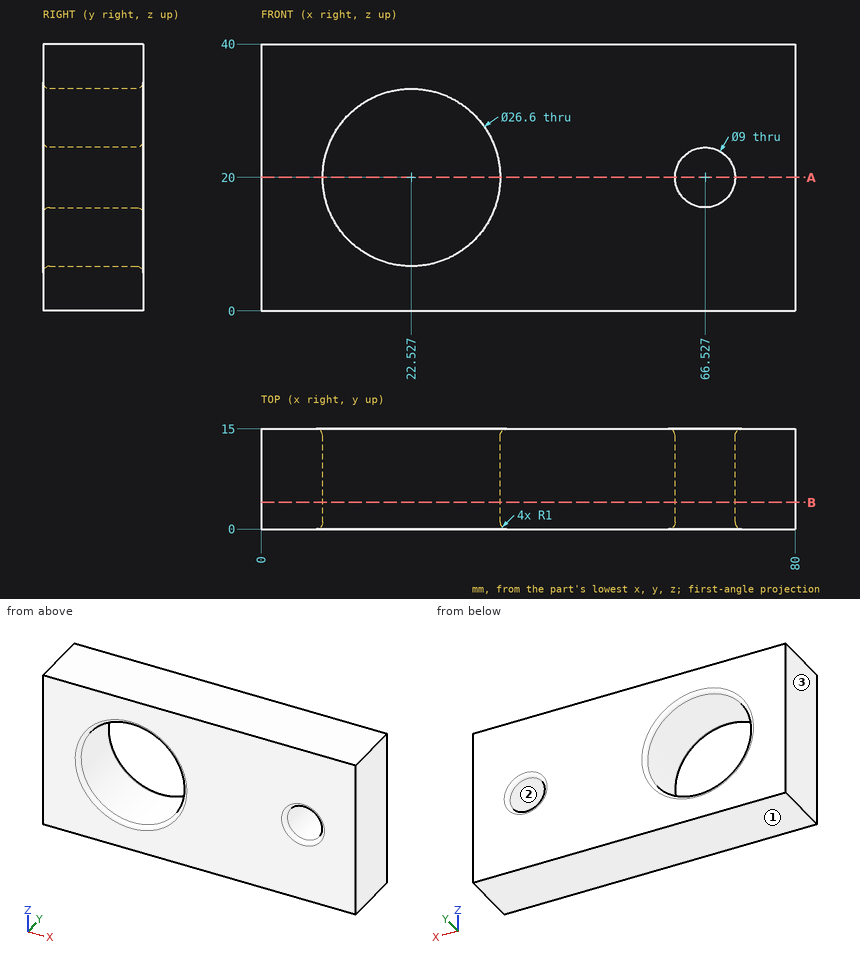
Geometry: see drawing. Coordinates: mm, zero at the bounding-box minimum. Round coordinates to 2 decimals unless told otherwise and drop trailing zeros. Write each loop counter-clockwise with the first axis right and the second up, starting at its lowest first coordinate (ties: lowest second). Pieces come first, ordered by that corner, then holes.
Item 1: Section query A-A (z = 20). Return loops of the section in (x, y), plus the area to 3 significant figures.
Item 2: Section query B-B (y = 4). Return loops of the section in (x, z).
Item 3: Mould query, pull axis Z, two halves, no side actions, for the marked faces 1, 2 and 3. Classes: +Z half, -Z half, draft (parallel to the pull), parting line (faces both ways), or undercut.
Item 4: Material intervals for L1, parallel to X at y = 7, z = 20; L2, parallel to X at y = 7, z = 18 (1 decimal); L3, parallel to Z at x = 16.5, y = 13 (1 decimal), sorted ascending.
Item 5: Pin query (flat end, axial travel): P1, Ø16, axis at x = 22.53, z = 20, coming from the -Y side. Return the tip coordinate at first contact, or that it passes through.
Completed:
1. outline: (0, 0) - (8.23, 0) arc R1 ccw to (9.23, 1) - (9.23, 14) arc R1 ccw to (8.23, 15) - (0, 15) - close; (35.83, 1) arc R1 ccw to (36.83, 0) - (61.03, 0) arc R1 ccw to (62.03, 1) - (62.03, 14) arc R1 ccw to (61.03, 15) - (36.83, 15) arc R1 ccw to (35.83, 14) - close; (71.03, 1) arc R1 ccw to (72.03, 0) - (80, 0) - (80, 15) - (72.03, 15) arc R1 ccw to (71.03, 14) - close
1. area: 664 mm2
2. outline: (0, 0) - (80, 0) - (80, 40) - (0, 40) - close; hole circle Ø26.6 at (22.53, 20); hole circle Ø9 at (66.53, 20)
3. face 1: -Z half
3. face 2: undercut
3. face 3: draft
4. L1: x = 0 to 9.23, 35.83 to 62.03, 71.03 to 80
4. L2: x = 0 to 9.4, 35.7 to 62.5, 70.6 to 80
4. L3: z = 0 to 8.1, 31.9 to 40
5. P1: passes through
